Read the model definition and answer for the solid it produces. Units are mm, in the model's axes. A direction names the side the tool comes from. Coordinates: 2 decimals unless noted, no trailing zeros. Order: outer loops, then holes, each group sorted by start corner. A loop starts at its lowest first (then second) coordinate and runs counter-clockwise, first axis right, second up. Notation, with made-up numbers: (57, -20) -> (85, -20) arc R24 cw to (85, 15) -> close; hole circle Ø4 at (66.25, -17.5). An arc over 180 degrees is marked (long way). Use CSV: the item, a comma, the result in double quotes.
```python
from build123d import *

# Parameters (mm, degrees)
F0_R      = 6.5
F0_W      = 34.999999702
F0_H      = 3
F0_H_2    = 0.3
F1_DEPTH  = 3
F2_DEPTH  = 9.5
F3_DEPTH  = 11.5
F5_DEPTH  = 3
F7_DEPTH  = 3
F8_R      = 1
F9_DEPTH  = 35.000999702
F11_DEPTH = 1
F13_DEPTH = 1
F14_SIZE  = 0.75
F15_W     = 1.8819853365
F15_H     = 1.731043148
F15_W_2   = 1.7636035271
F15_H_2   = 1.938064149
F16_DEPTH = 1
F18_DEPTH = 36.000999702
F19_R     = 1


# Not quite as in the source:
# - ends of sketch curves that miss each other by under 0.0002 mm in the source are joined
# - a feature names something its author has since deleted; it is built from what else it names


with BuildPart() as f1:
    # F0 (on Top) → F1 (new body)
    with BuildSketch(Plane.XY):
        Polygon((7.8607099131, 16.1003852367), (-9.6392899379, 16.1003852367), (-9.6392899379, -29.3996147633), (25.3607097641, -29.3996147633), (25.3607097641, 16.1003852367), align=None)
        with Locations((7.8607099131, -2.2867515218)):
            Circle(F0_R, mode=Mode.SUBTRACT)
        with Locations((7.8607099131, -31.1996147633)):
            Rectangle(F0_W, F0_H)
        Polygon((-9.6392899379, 19.1003852367), (-9.6392899379, 16.1003852367), (7.8607099131, 16.1003852367), (25.3607097641, 16.1003852367), (25.3607097641, 19.1003852367), (22.192974557, 19.1003852367), (3.3607097641, 19.1003852367), align=None)
        Polygon((-9.6392899379, 46.3003852367), (-9.6392899379, 43.3003852367), (-6.4715547308, 43.3003852367), (12.3607100621, 43.3003852367), (25.3607097641, 43.3003852367), (25.3607097641, 46.3003852367), align=None)
        with Locations((7.8607099131, -29.5496147633)):
            Rectangle(F0_W, F0_H_2)
        Polygon((16.0607097641, 38.1003852367), (25.3607097641, 38.1003852367), (25.3607097641, 43.3003852367), (12.3607100621, 43.3003852367), (12.3607100621, 35.3003852367), (12.3607100621, 34.5003852367), (7.8607097641, 34.5003852367), (7.8607100621, 33.9926332235), (8.7954637781, 33.9926332235), (16.0607097641, 33.9926332235), align=None)
        Polygon((-9.6392899379, 24.3003852367), (-9.6392899379, 19.1003852367), (3.3607097641, 19.1003852367), (3.3607097641, 27.1003852367), (3.3607097641, 27.9003852367), (7.8607100621, 27.9003852367), (7.8607100621, 28.4081372499), (6.9259563461, 28.4081372499), (-0.3392899379, 28.4081372499), (-0.3392899379, 24.3003852367), align=None)
        Polygon((6.9259563461, 34.5003852367), (6.9259563461, 28.4081372499), (7.8607097641, 28.4081372499), (7.8607100621, 33.9926332235), (7.8607100621, 34.5003852367), align=None)
        Polygon((7.8607100621, 28.4081372499), (7.8607100621, 27.9003852367), (8.7954637781, 27.9003852367), (8.7954637781, 33.9926332235), (7.8607097641, 33.9926332235), align=None)
        Polygon((-9.6392899379, 43.3003852367), (-9.6392899379, 24.3003852367), (-0.3392899379, 24.3003852367), (-0.3392899379, 28.4081372499), (6.9259563461, 28.4081372499), (6.9259563461, 34.5003852367), (7.8607100621, 34.5003852367), (12.3607100621, 34.5003852367), (12.3607100621, 35.3003852367), (12.3607100621, 43.3003852367), (-6.4715547308, 43.3003852367), align=None)
        Polygon((3.3607097641, 27.1003852367), (3.3607097641, 19.1003852367), (22.192974557, 19.1003852367), (25.3607097641, 19.1003852367), (25.3607097641, 38.1003852367), (16.0607097641, 38.1003852367), (16.0607097641, 33.9926332235), (8.7954637781, 33.9926332235), (8.7954637781, 27.9003852367), (7.8607100621, 27.9003852367), (3.3607097641, 27.9003852367), align=None)
    extrude(amount=-F1_DEPTH)

    # F0 (on Top) → F2 (join)
    with BuildSketch(Plane.XY):
        with Locations((7.8607099131, -31.1996147633)):
            Rectangle(F0_W, F0_H)
        Polygon((-9.6392899379, 19.1003852367), (-9.6392899379, 16.1003852367), (7.8607099131, 16.1003852367), (25.3607097641, 16.1003852367), (25.3607097641, 19.1003852367), (22.192974557, 19.1003852367), (3.3607097641, 19.1003852367), align=None)
    extrude(amount=F2_DEPTH)

    # F0 (on Top) → F3 (join)
    with BuildSketch(Plane.XY):
        Polygon((-9.6392899379, 46.3003852367), (-9.6392899379, 43.3003852367), (-6.4715547308, 43.3003852367), (12.3607100621, 43.3003852367), (25.3607097641, 43.3003852367), (25.3607097641, 46.3003852367), align=None)
        Polygon((-9.6392899379, 24.3003852367), (-9.6392899379, 19.1003852367), (3.3607097641, 19.1003852367), (3.3607097641, 27.1003852367), (3.3607097641, 27.9003852367), (7.8607100621, 27.9003852367), (7.8607100621, 28.4081372499), (6.9259563461, 28.4081372499), (-0.3392899379, 28.4081372499), (-0.3392899379, 24.3003852367), align=None)
        Polygon((7.8607100621, 28.4081372499), (7.8607100621, 27.9003852367), (8.7954637781, 27.9003852367), (8.7954637781, 33.9926332235), (7.8607097641, 33.9926332235), align=None)
        Polygon((6.9259563461, 34.5003852367), (6.9259563461, 28.4081372499), (7.8607097641, 28.4081372499), (7.8607100621, 33.9926332235), (7.8607100621, 34.5003852367), align=None)
        Polygon((16.0607097641, 38.1003852367), (25.3607097641, 38.1003852367), (25.3607097641, 43.3003852367), (12.3607100621, 43.3003852367), (12.3607100621, 35.3003852367), (12.3607100621, 34.5003852367), (7.8607097641, 34.5003852367), (7.8607100621, 33.9926332235), (8.7954637781, 33.9926332235), (16.0607097641, 33.9926332235), align=None)
    extrude(amount=F3_DEPTH)

    # F4 (on face) → F5 (join)
    with BuildSketch(Plane.YZ.offset(25.3607097641)):
        Polygon((-32.6996147633, -3), (46.3003852367, -3), (46.3003852367, 11.5), (38.1003852367, 11.5), (38.1003852367, 0), (19.1003852367, 0), (19.1003852367, 9.5), (16.1003852367, 9.5), (16.1003852367, 0), (-29.6996147633, 0), (-29.6996147633, 9.5), (-32.6996147633, 9.5), align=None)
        with BuildLine():
            Line((46.3003852367, 11.5), (46.3003852367, -3))
            Line((46.3003852367, -3), (60.2135883006, 16.6053474951))
            ThreePointArc((60.2135883006, 16.6053474951), (54.0324103863, 15.4756413664), (52.7478740756, 21.6265082006))
            Line((52.7478740756, 21.6265082006), (46.3003852367, 11.5))
        make_face()
        with BuildLine():
            ThreePointArc((52.7478740756, 21.6265082006), (54.0324103863, 15.4756413664), (60.2135883006, 16.6053474951))
            ThreePointArc((60.2135883006, 16.6053474951), (60.8312132136, 17.8429507129), (61.0437823534, 19.2096754909))
            ThreePointArc((61.0437823534, 19.2096754909), (57.8024349564, 23.5300682537), (52.7478740756, 21.6265082006))
        make_face()
        with BuildLine():
            Line((-41.5630528886, -1.9133363436), (-32.6996147633, -3))
            Line((-32.6996147633, -3), (-32.6996147633, 9.5))
            Line((-32.6996147633, 9.5), (-42.2056278, 6.8929759665))
            ThreePointArc((-42.2056278, 6.8929759665), (-38.2865124349, 6.1313346687), (-36.5154499114, 2.5532206055))
            ThreePointArc((-36.5154499114, 2.5532206055), (-38.0333544566, -0.8168100619), (-41.5630528886, -1.9133363436))
        make_face()
        with BuildLine():
            ThreePointArc((-42.2056278, 6.8929759665), (-45.503517949, 2.2257373389), (-41.5630528886, -1.9133363436))
            ThreePointArc((-41.5630528886, -1.9133363436), (-38.0333544566, -0.8168100619), (-36.5154499114, 2.5532206055))
            ThreePointArc((-36.5154499114, 2.5532206055), (-38.2865124349, 6.1313346687), (-42.2056278, 6.8929759665))
        make_face()
    extrude(amount=-F5_DEPTH)

    # F6 (on face) → F7 (join)
    with BuildSketch(Plane(origin=(-9.6392899379, 0, 0), x_dir=(0, -1, 0), z_dir=(-1, 0, 0))):
        with BuildLine():
            Line((-60.2135883006, 16.6053474951), (-46.3003852367, -3))
            Line((-46.3003852367, -3), (-46.3003852367, 11.5))
            Line((-46.3003852367, 11.5), (-52.7478740756, 21.6265082006))
            ThreePointArc((-52.7478740756, 21.6265082006), (-59.0551543205, 22.9437096154), (-60.2135883006, 16.6053474951))
        make_face()
        Polygon((-46.3003852367, 11.5), (-46.3003852367, -3), (32.6996147633, -3), (32.6996147633, 9.5), (29.6996147633, 9.5), (29.6996147633, 0), (-16.1003852367, 0), (-16.1003852367, 9.5), (-19.1003852367, 9.5), (-19.1003852367, 11.5), (-24.3003852367, 11.5), (-24.3003852367, 0), (-43.3003852367, 0), (-43.3003852367, 11.5), align=None)
        with BuildLine():
            Line((32.6996147633, 9.5), (32.6996147633, -3))
            Line((32.6996147633, -3), (41.5630528886, -1.9133363436))
            ThreePointArc((41.5630528886, -1.9133363436), (45.503517949, 2.2257373389), (42.2056278, 6.8929759665))
            Line((42.2056278, 6.8929759665), (32.6996147633, 9.5))
        make_face()
    extrude(amount=-F7_DEPTH)

    # F8 (on face) → F9 (cut, through all)
    with BuildSketch(Plane(origin=(-9.6392899379, 0, 0), x_dir=(0, -1, 0), z_dir=(-1, 0, 0))):
        with Locations((-56.5437823534, 19.2096754909)):
            Circle(F8_R)
        with Locations((41.0154499114, 2.5532206055)):
            Circle(F8_R)
    extrude(amount=-F9_DEPTH, mode=Mode.SUBTRACT)

    # F10 (on face) → F11 (join)
    with BuildSketch(Plane.YZ.offset(25.3607097641)):
        Polygon((39.4906885922, 7.75), (38.1003852367, 7.75), (38.1003852367, 3.75), (39.4906885922, 3.75), (39.4906885922, 5.75), align=None)
        Polygon((38.1003852367, 3.75), (38.1003852367, 7.75), (37.4906885922, 7.75), (37.4906885922, 5.75), (37.4906885922, 3.75), align=None)
    extrude(amount=F11_DEPTH)

    # F12 (on face) → F13 (join)
    with BuildSketch(Plane(origin=(-9.6392899379, 0, 0), x_dir=(0, -1, 0), z_dir=(-1, 0, 0))):
        Polygon((-22.9083076119, 7.75), (-24.3003852367, 7.75), (-24.3003852367, 3.75), (-22.9083076119, 3.75), (-22.9083076119, 5.75), align=None)
        Polygon((-24.9083076119, 7.75), (-24.9083076119, 5.75), (-24.9083076119, 3.75), (-24.3003852367, 3.75), (-24.3003852367, 7.75), align=None)
    extrude(amount=F13_DEPTH)

    # F14
    f14_edges = [f1.edges().sort_by_distance(p)[0] for p in [
        (-10.63929, 24.908308, 5.75),
        (-10.63929, 22.908308, 5.75),
        (-10.63929, 23.908308, 7.75),
        (-10.63929, 23.908308, 3.75),
        (26.36071, 38.490689, 7.75),
        (26.36071, 37.490689, 5.75),
        (26.36071, 38.490689, 3.75),
        (26.36071, 39.490689, 5.75),
    ]]
    chamfer(f14_edges, length=F14_SIZE)

    # F15 (on face) → F16 (join)
    with BuildSketch(Plane.XY.offset(11.5)):
        with Locations((11.4197173938, 35.3659068108)):
            Rectangle(F15_W, F15_H)
        with Locations((4.2425115276, 26.9313531622)):
            Rectangle(F15_W_2, F15_H_2)
    extrude(amount=-F16_DEPTH)

    # F17 (on face) → F18 (cut, through all)
    with BuildSketch(Plane(origin=(-9.6392899379, 0, 0), x_dir=(0, -1, 0), z_dir=(-1, 0, 0))):
        with BuildLine():
            Line((-56.1974216606, 10.9460940352), (-46.3003852367, -3))
            Line((-46.3003852367, -3), (-32.2360508144, -3))
            add(Edge.make_bspline(
                [(-56.1974216606, 10.9460940352), (-49.7821666885, 1.9062415714), (-46.3003852367, -3), (-32.2360508144, -3)],
                knots=[0, 0, 0, 0, 27.7243725207, 27.7243725207, 27.7243725207, 27.7243725207], degree=3))
        make_face()
    extrude(amount=-F18_DEPTH, mode=Mode.SUBTRACT)

    # F19
    f19_edges = [f1.edges().sort_by_distance(p)[0] for p in [
        (5.124313, 25.962321, 11),
        (10.478725, 36.231428, 11),
    ]]
    fillet(f19_edges, radius=F19_R)


solid = f1.part
```
Item 1: Find section B-B, the plane y = -13. Give the vertices of the cut face in (x, z), then the cut area to 3 significant figures.
Return value:
outline,"(-9.64, -3) -> (25.36, -3) -> (25.36, 0) -> (-9.64, 0) -> close"
area,"105 mm^2"
Item 2: A tool of negligible diameter and unlimited length cuts with its end or side. For faces 1 (the flat face through (8, -31, 9.5)), 2 (the flat face through (8, -12, 0)), 3 (the flat face through (10, 34.5, 6)), from which of +Z, -Z, +X, -X, +Y, -Y can it reach the whole face along a straight path? Write none if from no direction.
Return value:
face 1,"+Z, +X, -X, -Y"
face 2,"+Z, +X, -X"
face 3,"-X"
Item 3: Straight lines are drawn through the part: line 1 along Y through (x, z) = (1, 0.5); line 2 along Y through (x, z) = (14.5, 1.75); line 3 along Z through (x, y) = (4, 26.5). For each, find the intervals that lie inside material, in ascending order.
Return value:
line 1,"y = -32.7 to -29.7, 16.1 to 28.41, 43.3 to 46.3"
line 2,"y = -32.7 to -29.7, 16.1 to 19.1, 33.99 to 46.3"
line 3,"z = -3 to 0, 10.5 to 11.5"
Item 4: Find section C-C, the plane y = 3. Give the vertices of the cut face in (x, z), then the cut area to 3 significant figures.
Return value:
outline,"(-9.64, -3) -> (4.08, -3) -> (4.08, 0) -> (-9.64, 0) -> close; (11.64, -3) -> (25.36, -3) -> (25.36, 0) -> (11.64, 0) -> close"
area,"82.3 mm^2"
Item 5: Find section A-A, the plane y = -35. Give the vertices of the cut face in (x, z), then the cut area to 3 significant figures.
Return value:
outline,"(-9.64, -2.72) -> (-6.64, -2.72) -> (-6.64, 8.87) -> (-9.64, 8.87) -> close; (22.36, -2.72) -> (25.36, -2.72) -> (25.36, 8.87) -> (22.36, 8.87) -> close"
area,"69.5 mm^2"
Item 6: The mould has two halves that part along Y. Classify faces 4 (the flat face through (12, 33.993, 6)), 5 (the flat face through (22.361, 54, 15)), 6 (the cylindrical face through (-8.16, -41.97, 2.85)), 7 (the flat face through (23.882, -37.386, 8.215)): +Y half, -Y half, draft (parallel to the pull), parting line (faces both ways), or undercut.
Return value:
face 4,"undercut"
face 5,"draft"
face 6,"undercut"
face 7,"-Y half"
Item 7: Each of these flat-tipped pins is pushed along its axis until it touches: P1, Ø10.5, axis at x = 7, z = 5, coming from the -Y side; P2, Ø7, axis at y = 25.5, z = 8.5, coming from the +X side; P3, Ø3, axis at x = 5, y = 29.5, coming from the +Z side. Where does it stop, or does it pass through?
Return value:
P1,"stops at y = -32.7"
P2,"stops at x = 8.8"
P3,"stops at z = 11.5"
